Part model, mm, in its own coordinate system. Face numbers are marked on the shaded views. A direction names the side the tool comes from. Round coordinates to 2 decimals unless told otherwise and drop trailing zeros. Loops run counter-clockwise (first coordinate to the right, second up) from the corner with the lowest first, then second, coordinate; pieces in that order, holes last.
(1) Tool access for the marked faces 1 and 2: list every direction of +Z, -Z, +X, -X, +Y, -Y with a clear straight run to the whole face (end or side of a thin tool).
(2) Cut at C-C on x = 8. List the corners of the cut face in (y, z).
(3) Cut at D-D on z = -20. List the corners of the cut face in (x, y), then the cut area to 3 significant figures.
(4) Cut at B-B on y = -15.5. Count the separate pieces of the cut face and the enclosed holes in it, then the cut area to 3 significant figures.
(5) Flat gauge pins, fed straight in: pin 1 (3 mm diameter, centred on y = -18, z = 28.5, fed in from +X); pin 2 (8 mm diameter, centred on x = 5.5, z = 9, fed in from +Y); pin 3 (1.2 mm diameter, centred on y = -10.5, z = 31, fed in from -X). Where does each tip first touch, or does it go through?
(6) Mould opens along Y. For the marked faces 3, 4, 5 and 6 say: +Y half, -Y half, draft (parallel to the pull), parting line (faces both ways), or undercut.
(7) Cut at A-A on z = 31.5. List the corners of the cut face in (x, y).
(8) Probe probe 1 along Y at (x, z) = (0.85, 15.5); probe 2 along Z at (x, y) = (3.95, 15.5) (3 decimals); probe 3 along X at (y, z) = (10, -24). List the from-to ranges inside material, lowest first.
from build123d import *

# Parameters (mm, degrees)
CROQUIS1_W              = 47
CROQUIS1_H              = 47
CROQUIS1_R              = 1.65
SALIENTE_EXTRUIR1_DEPTH = 5.5
CORTAR_EXTRUIR1_DEPTH   = 2.35
CROQUIS7_R              = 12.35
CORTAR_EXTRUIR2_DEPTH   = 5.5
CROQUIS8_R              = 1.7
CORTAR_EXTRUIR3_DEPTH   = 5.5
CROQUIS9_W              = 49.5
CROQUIS9_H              = 49.5
CROQUIS9_W_2            = 43.5
CROQUIS9_H_2            = 43.5
SALIENTE_EXTRUIR2_DEPTH = 25.5
CROQUIS10_R             = 10
SALIENTE_EXTRUIR3_DEPTH = 15
CORTAR_EXTRUIR4_REACH   = 73.141
REDONDEO1_R             = 10
CROQUIS13_R             = 1.7
SALIENTE_EXTRUIR5_DEPTH = 12.1
CORTAR_EXTRUIR5_REACH   = 73.141
CROQUIS14_W             = 6
CROQUIS14_H             = 4.1
CHAFL_N1_SIZE           = 3
CROQUIS15_W             = 7
CROQUIS15_H             = 3
SALIENTE_EXTRUIR6_DEPTH = 10
CORTAR_EXTRUIR6_REACH   = 73.157
CROQUIS16_R             = 1.7
REDONDEO2_R             = 2
REDONDEO4_R             = 2
CROQUIS18_R             = 3.25
CORTAR_EXTRUIR7_DEPTH   = 2.5


# Some blends are built 0.0001 mm under size
with BuildPart() as part:
    # Croquis1 → Saliente-Extruir1 (new body)
    with BuildSketch(Plane(origin=(0, 0, 0), x_dir=(0, 0, -1), z_dir=(1, 0, 0))):
        Rectangle(CROQUIS1_W, CROQUIS1_H)
        with Locations((-15.5, 15.5)):
            Circle(CROQUIS1_R, mode=Mode.SUBTRACT)
        with Locations((15.5, 15.5)):
            Circle(CROQUIS1_R, mode=Mode.SUBTRACT)
        with Locations((15.5, -15.5)):
            Circle(CROQUIS1_R, mode=Mode.SUBTRACT)
        with Locations((-15.5, -15.5)):
            Circle(CROQUIS1_R, mode=Mode.SUBTRACT)
    extrude(amount=SALIENTE_EXTRUIR1_DEPTH)

    # Croquis2 → Cortar-Extruir1 (cut)
    with BuildSketch(Plane(origin=(5.5, 0, 0), x_dir=(0, 0, -1), z_dir=(1, 0, 0))):
        Polygon((0, 13.968911087), (2.625, 15.484455543), (2.625, 18.515544457), (0, 20.031088913), (-2.625, 18.515544457), (-2.625, 15.484455543), align=None)
        Polygon((14.722431864, -11.531088913), (17.347431864, -10.015544457), (17.347431864, -6.984455543), (14.722431864, -5.468911087), (12.097431864, -6.984455543), (12.097431864, -10.015544457), align=None)
        Polygon((-17.347431864, -6.984455543), (-17.347431864, -10.015544457), (-14.722431864, -11.531088913), (-12.097431864, -10.015544457), (-12.097431864, -6.984455543), (-14.722431864, -5.468911087), align=None)
    extrude(amount=-CORTAR_EXTRUIR1_DEPTH, mode=Mode.SUBTRACT)

    # Croquis7 → Cortar-Extruir2 (cut)
    with BuildSketch(Plane(origin=(5.5, 0, 0), x_dir=(0, 0, -1), z_dir=(1, 0, 0))):
        Circle(CROQUIS7_R)
    extrude(amount=-CORTAR_EXTRUIR2_DEPTH, mode=Mode.SUBTRACT)

    # Croquis8 → Cortar-Extruir3 (cut)
    with BuildSketch(Plane(origin=(5.5, 0, 0), x_dir=(0, 0, -1), z_dir=(1, 0, 0))):
        with Locations((0, 17)):
            Circle(CROQUIS8_R)
        with Locations((14.722431864, -8.5)):
            Circle(CROQUIS8_R)
        with Locations((-14.722431864, -8.5)):
            Circle(CROQUIS8_R)
    extrude(amount=-CORTAR_EXTRUIR3_DEPTH, mode=Mode.SUBTRACT)

    # Croquis9 → Saliente-Extruir2 (add)
    with BuildSketch(Plane(origin=(0, 0, 0), x_dir=(0, 0, -1), z_dir=(1, 0, 0))):
        Rectangle(CROQUIS9_W, CROQUIS9_H)
        Rectangle(CROQUIS9_W_2, CROQUIS9_H_2, mode=Mode.SUBTRACT)
    extrude(amount=SALIENTE_EXTRUIR2_DEPTH)

    # Croquis10 → Saliente-Extruir3 (add)
    with BuildSketch(Plane(origin=(0, 21.75, 0), x_dir=(1, 0, 0), z_dir=(0, 1, 0))):
        with Locations(Location((25.5, 0, 0), (0, 0, 270))):
            Circle(CROQUIS10_R)
    saliente_extruir3 = extrude(amount=SALIENTE_EXTRUIR3_DEPTH)

    # Simetría1: Saliente-Extruir3 across plane
    add(saliente_extruir3.mirror(Plane.ZX))

    # Cortar-Extruir4: up to this face of the body (flat: up to its plane)
    cortar_extruir4_end = Plane(part.part.faces().sort_by_distance((12.75, 0, 24.75))[0])
    # Croquis11 → Cortar-Extruir4 (cut, up to the picked face)
    with BuildSketch(Plane(origin=(0, 0, -24.75), x_dir=(-1, 0, 0), z_dir=(0, 0, -1)), mode=Mode.PRIVATE) as cortar_extruir4_sk1:
        with BuildLine():
            Line((-7, -13.75), (-7, 13.75))
            ThreePointArc((-7, 13.75), (-8.171572875, 16.578427125), (-11, 17.75))
            Line((-11, 17.75), (-14.5, 17.75))
            ThreePointArc((-14.5, 17.75), (-17.328427125, 16.578427125), (-18.5, 13.75))
            Line((-18.5, 13.75), (-18.5, -13.75))
            ThreePointArc((-18.5, -13.75), (-17.328427125, -16.578427125), (-14.5, -17.75))
            Line((-14.5, -17.75), (-11, -17.75))
            ThreePointArc((-11, -17.75), (-8.171572875, -16.578427125), (-7, -13.75))
        make_face()
    cortar_extruir4_tool1 = split(extrude(cortar_extruir4_sk1.sketch, amount=-CORTAR_EXTRUIR4_REACH, mode=Mode.PRIVATE), bisect_by=cortar_extruir4_end, keep=Keep.BOTH, mode=Mode.PRIVATE)
    add(cortar_extruir4_tool1.solids().sort_by(Axis((12.75, 0, -24.75), (0, 0, 1)))[0], mode=Mode.SUBTRACT)

    # Redondeo1
    # the kernel refuses this fillet: 10 mm, written as the material it adds along each edge
    with BuildSketch(Plane(origin=(25.5, 21.75, 10), x_dir=(0, 0, 1), z_dir=(0, 1, 0)), Plane(origin=(25.5, 24.75, -10), x_dir=(0, 0, -1), z_dir=(0, -1, 0))) as redondeo1_piece_1:
        with BuildLine():
            CenterArc((7.320508076, 10), REDONDEO1_R, 210, 60)
            ThreePointArc((-1.339745962, 5), (-0.340741737, 2.588190451), (0, 0))
            Line((0, 0), (7.320508076, 0))
        make_face()
    extrude(amount=3)
    with BuildSketch(Plane(origin=(25.5, -24.75, -10), x_dir=(0, 0, -1), z_dir=(0, 1, 0))) as redondeo1_piece_2:
        with BuildLine():
            CenterArc((7.320508076, -10), REDONDEO1_R, 90, 60)
            ThreePointArc((-1.339745962, -5), (-0.340741737, -2.588190451), (0, 0))
            Line((0, 0), (7.320508076, 0))
        make_face()
    extrude(amount=3)
    with BuildSketch(Plane(origin=(25.5, -21.75, 10), x_dir=(0.9659258262890682, 0, -0.2588190451025209), z_dir=(0, -1, 0))) as redondeo1_piece_3:
        with BuildLine():
            CenterArc((7.764571353, 9.659258263), REDONDEO1_R, 195, 60)
            Line((-1.89468691, 7.071067812), (0, 0))
            ThreePointArc((0, 0), (2.588190451, 0.340741737), (5.176380902, 0))
        make_face()
    extrude(amount=3)

    # Croquis13 → Saliente-Extruir5 (add)
    with BuildSketch(Plane.XZ.offset(20.75)):
        Polygon((28.5, -35.75), (28.5, -24.75), (22.5, -24.75), (22.5, -35.75), (23.977414586, -35.75), (27.022585414, -35.75), align=None)
        with Locations(Location((25.5, -31.5, 0), (0, 0, 270))):
            Circle(CROQUIS13_R, mode=Mode.SUBTRACT)
    saliente_extruir5 = extrude(amount=-SALIENTE_EXTRUIR5_DEPTH)

    # Cortar-Extruir5: up to this face of the body (flat: up to its plane)
    cortar_extruir5_end = Plane(part.part.faces().sort_by_distance((25.5, -14.7, -35.75))[0])
    # Croquis14 → Cortar-Extruir5 (cut, up to the picked face)
    with BuildSketch(Plane(origin=(0, 0, -24.75), x_dir=(-1, 0, 0), z_dir=(0, 0, -1)), mode=Mode.PRIVATE) as cortar_extruir5_sk1:
        with Locations((-25.5, -14.7)):
            Rectangle(CROQUIS14_W, CROQUIS14_H)
    cortar_extruir5_tool1 = split(extrude(cortar_extruir5_sk1.sketch, amount=CORTAR_EXTRUIR5_REACH, mode=Mode.PRIVATE), bisect_by=cortar_extruir5_end, keep=Keep.BOTH, mode=Mode.PRIVATE)
    cortar_extruir5 = cortar_extruir5_tool1.solids().sort_by(Axis((25.5, -14.7, -24.75), (0, 0, -1)))[0]
    add(cortar_extruir5, mode=Mode.SUBTRACT)

    # Simetría2: Saliente-Extruir5, Cortar-Extruir5 across plane
    add(saliente_extruir5.mirror(Plane.XY))
    add(cortar_extruir5.mirror(Plane.XY), mode=Mode.SUBTRACT)

    # Chaflán1
    chafl_n1_edges = [part.edges().sort_by_distance(p)[0] for p in [
        (25.5, -18.75, -24.75),
        (22.5, -10.65, -24.75),
        (22.5, -18.75, -24.75),
        (25.5, -10.65, -24.75),
        (25.5, -10.65, 24.75),
        (22.5, -10.65, 24.75),
        (22.5, -18.75, 24.75),
        (25.5, -18.75, 24.75),
    ]]
    chamfer(chafl_n1_edges, length=CHAFL_N1_SIZE - 0.0001)  # a hair under: the kernel refuses the full size

    # Croquis15 → Saliente-Extruir6 (add)
    with BuildSketch(Plane(origin=(0, 0, -24.75), x_dir=(-1, 0, 0), z_dir=(0, 0, -1))):
        with Locations((-3.5, 12)):
            Rectangle(CROQUIS15_W, CROQUIS15_H)
        with Locations((-3.5, -12)):
            Rectangle(CROQUIS15_W, CROQUIS15_H)
    extrude(amount=SALIENTE_EXTRUIR6_DEPTH)

    # Cortar-Extruir6: up to this face of the body (flat: up to its plane)
    cortar_extruir6_end = Plane(part.part.faces().sort_by_distance((3.5, 13.5, -29.75))[0])
    # Croquis16 → Cortar-Extruir6 (cut, up to the picked face)
    with BuildSketch(Plane.XZ.offset(13.5), mode=Mode.PRIVATE) as cortar_extruir6_sk1:
        with Locations((3.5, -29.75)):
            Circle(CROQUIS16_R)
    cortar_extruir6_tool1 = split(extrude(cortar_extruir6_sk1.sketch, amount=-CORTAR_EXTRUIR6_REACH, mode=Mode.PRIVATE), bisect_by=cortar_extruir6_end, keep=Keep.BOTH, mode=Mode.PRIVATE)
    add(cortar_extruir6_tool1.solids().sort_by(Axis((3.5, -13.5, -29.75), (0, 1, 0)))[0], mode=Mode.SUBTRACT)

    # Redondeo2
    redondeo2_edges = [part.edges().sort_by_distance(p)[0] for p in [
        (0, 12, -34.75),
        (7, 12, -34.75),
        (0, -12, -34.75),
        (7, -12, -34.75),
    ]]
    fillet(redondeo2_edges, radius=REDONDEO2_R)

    # Redondeo4
    redondeo4_edges = [part.edges().sort_by_distance(p)[0] for p in [
        (28.5, -10.65, -35.75),
        (22.5, -10.65, -35.75),
        (28.5, -18.75, -35.75),
        (22.5, -18.75, -35.75),
        (22.5, -10.65, 35.75),
        (28.5, -10.65, 35.75),
        (22.5, -18.75, 35.75),
        (28.5, -18.75, 35.75),
    ]]
    fillet(redondeo4_edges, radius=REDONDEO4_R)

    # Croquis18 → Cortar-Extruir7 (cut)
    with BuildSketch(Plane.ZY):
        with Locations((-15.5, 15.5)):
            Circle(CROQUIS18_R)
        with Locations((15.5, 15.5)):
            Circle(CROQUIS18_R)
        with Locations((15.5, -15.5)):
            Circle(CROQUIS18_R)
        with Locations((-15.5, -15.5)):
            Circle(CROQUIS18_R)
    extrude(amount=-CORTAR_EXTRUIR7_DEPTH, mode=Mode.SUBTRACT)


solid = part.part
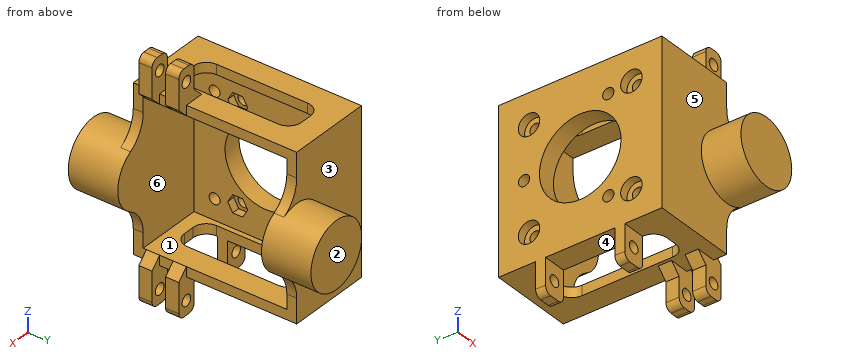
Final values:
1. face 1: +X
1. face 2: +Z, -Z, +X, -X, +Y
2. outline: (-24.75, -24.75) - (-16.4, -24.75) - (-16.4, -21.75) - (-21.75, -21.75) - (-21.75, 21.75) - (-16.4, 21.75) - (-16.4, 24.75) - (-24.75, 24.75) - close; (16.4, -24.75) - (24.75, -24.75) - (24.75, 24.75) - (16.4, 24.75) - (16.4, 21.75) - (21.75, 21.75) - (21.75, -21.75) - (16.4, -21.75) - close
3. outline: (0, -24.75) - (25.5, -24.75) - (25.5, -21.75) - (5.5, -21.75) - (5.5, 21.75) - (25.5, 21.75) - (25.5, 24.75) - (0, 24.75) - close
3. area: 392 mm2
4. separate pieces: 5
4. enclosed holes: 0
4. area: 276 mm2
5. pin 1: stops at x = 28.5
5. pin 2: stops at y = 24.75
5. pin 3: stops at x = 22.5
6. face 3: +Y half
6. face 4: undercut
6. face 5: -Y half
6. face 6: undercut
7. outline: (22.5, -20.75) - (23.8, -20.75) - (23.8, -16.75) - (22.5, -16.75) - close; (22.5, -12.65) - (23.8, -12.65) - (23.8, -8.65) - (22.5, -8.65) - close; (27.2, -20.75) - (28.5, -20.75) - (28.5, -16.75) - (27.2, -16.75) - close; (27.2, -12.65) - (28.5, -12.65) - (28.5, -8.65) - (27.2, -8.65) - close
8. probe 1: y = -24.75 to -18.75, -12.25 to -10.01, -6.99 to 12.25, 18.75 to 24.75
8. probe 2: z = -24.75 to -17.15, -13.85 to -2.625, 2.625 to 13.85, 17.15 to 24.75
8. probe 3: x = 0 to 7, 18.5 to 25.5
